from build123d import *

# Parameters (mm, degrees)
SKETCH2_W               = 500
SKETCH2_H               = 12.5
BOSS_EXTRUDE1_DEPTH     = 500
SKETCH6_R               = 6.25
BOSS_EXTRUDE3_DEPTH     = 500
BOSS_EXTRUDE4_DEPTH     = 500
CUT_EXTRUDE2_DEPTH      = 674.624176563
CUT_EXTRUDE2_DEPTH_BACK = 674.624176563
SKETCH9_R               = 2.5
CUT_EXTRUDE3_DEPTH      = 20
INTERSECT3_START        = -357.972808076
INTERSECT3_DEPTH        = 351.722808076


# Read off the part's stored shape, not the designer's step: Intersect3
with BuildPart() as part:
    # Sketch2 → Boss-Extrude1 (new body)
    with BuildSketch(Plane(origin=(-134.375, 134.375, 0), x_dir=(0, 0, 1), z_dir=(0.7071067811865464, -0.7071067811865488, 0))):
        with Locations((0, 190.034947444)):
            Rectangle(SKETCH2_W, SKETCH2_H)
    extrude(amount=BOSS_EXTRUDE1_DEPTH)

    # Sketch6 → Boss-Extrude3 (add)
    with BuildSketch(Plane.XY.offset(250)):
        with Locations((-268.75, 0)):
            Circle(SKETCH6_R)
    extrude(amount=-BOSS_EXTRUDE3_DEPTH)

    # Sketch7 → Boss-Extrude4 (add)
    with BuildSketch(Plane.XY.offset(250)):
        Polygon((-268.75, 6.25), (-262.5, 6.25), (91.053390593, -347.303390593), (89.222807976, -349.133973211), align=None)
    extrude(amount=-BOSS_EXTRUDE4_DEPTH)

    # Sketch8 → Cut-Extrude2 (cut, two sides: drawn at the far end of the back side and taken through both)
    with BuildSketch(Plane.XY.offset(250).offset(-CUT_EXTRUDE2_DEPTH_BACK)):
        with BuildLine():
            Line((-268.75, 6.25), (-263.442130557, 9.619585215))
            Line((-263.442130557, 9.619585215), (-256.25, 0))
            add(Edge.make_bspline(
                [(-268.75, 6.25), (-263.635709853, 6.25), (-259.544039229, 3.294039229), (-256.25, 0)],
                knots=[0, 0, 0, 0, 1, 1, 1, 1], degree=3))
        make_face()
    extrude(amount=CUT_EXTRUDE2_DEPTH + CUT_EXTRUDE2_DEPTH_BACK, mode=Mode.SUBTRACT)

    # Sketch9 → Cut-Extrude3 (cut)
    with BuildSketch(Plane.XY.offset(250)):
        with Locations((-268.75, 0)):
            Circle(SKETCH9_R)
    cut_extrude3 = extrude(amount=-CUT_EXTRUDE3_DEPTH, mode=Mode.SUBTRACT)

    # Mirror2: Cut-Extrude3 across plane
    add(cut_extrude3.mirror(Plane.XY), mode=Mode.SUBTRACT)

    # Intersect3 outline → Intersect3 (cut)
    with BuildSketch(Plane(origin=(0, 0, 0), x_dir=(1, 0, 0), z_dir=(0, 1, 0)).offset(INTERSECT3_START)):
        Polygon((-250, 250), (0, 0), (-250, -250), (93, -250), (93, 250), align=None)
    extrude(amount=INTERSECT3_DEPTH, mode=Mode.SUBTRACT)


solid = part.part
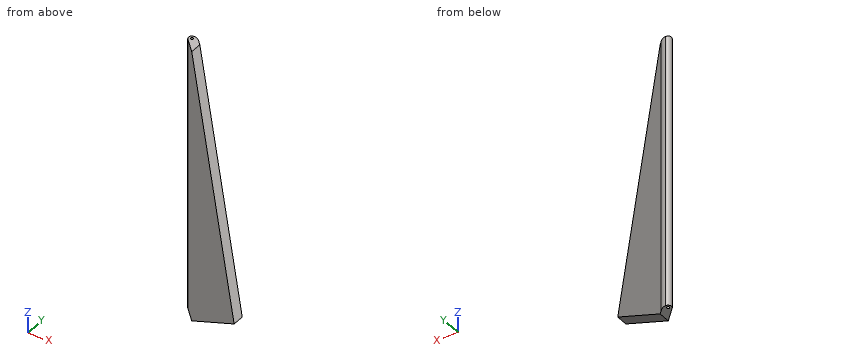
Could you check a few things on this model? Use its own coordinates, in mm. Give positions to 0.01 mm unless a question says otherwise; leave off trailing zeros. Write each loop counter-clockwise with the first axis right and the second up, starting at its lowest first coordinate (ties: lowest second). Pieces come first, ordered by that corner, then holes. Notation, with made-up numbers: (56.5, 46) - (84.5, 46) arc R20 cw to (84.5, 76) - close; hole circle Ø7 at (51, 54.25). An arc over 180 degrees is marked (long way). Use CSV: the item, a comma, the result in double quotes. Start each with the question number.
Item 1: I'm going to push flat-ended pins straight in: pin 1 (6 mm diameter, centred on y = -95, z = -34, fed in from -X); pin 2 (3 mm diameter, centred on x = -268.75, y = 0, fed in from -Z); pin 3 (2 mm diameter, centred on x = -234, z = 3, fed in from -Y). Where does each tip first touch, or does it pass through?
Item 2: I want a section at B-B, the plane y = -103.5. Please give me the cut outline in (x, z).
Item 3: I want a section at A-A, the plane x = -203. Please give me the cut outline in (y, z).
Item 4: If I drill on line 1 along Y through (x, z) = (-268.75, -241.5); line 2 along Y through (x, z) = (-32.5, 7); line 3 along Z through (x, y) = (-23.5, -250.5), over which ranges is the centre line in solid material (lowest first)?
Findings:
1,pin 1,"stops at x = -185.59"
1,pin 2,"stops at z = -230"
1,pin 3,"stops at y = -44.59"
2,outline,"(-174.09, -174.09) - (-152.75, -152.75) - (-152.75, 152.75) - (-174.09, 174.09) - close"
3,outline,"(-74.59, -203) - (-53.25, -203) - (-53.25, 203) - (-74.59, 203) - close"
4,line 1,"y = -8.84 to -2.5, 2.5 to 6.25"
4,line 2,"y = -245.09 to -223.75"
4,line 3,"z = -23.5 to 23.5"
